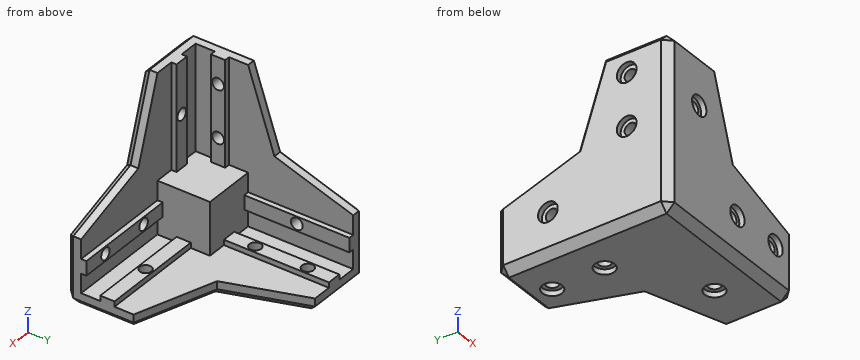
```python
from build123d import *

# Parameters (mm, degrees)
F1_DEPTH  = 6
F3_DEPTH  = 20
F5_DEPTH  = 40
F7_DEPTH  = 60
F9_DEPTH  = 2
F11_DEPTH = 2
F13_DEPTH = 2
F14_R     = 2.25
F15_DEPTH = 8
F16_R     = 2.25
F17_DEPTH = 8
F18_R     = 2.25
F19_DEPTH = 8
F20_R     = 3.75
F21_DEPTH = 2
F22_R     = 3.75
F23_DEPTH = 2
F24_R     = 3.75
F25_DEPTH = 2
F26_W     = 20
F26_H     = 20
F27_DEPTH = 20
F29_DEPTH = 6
F31_DEPTH = 6
F33_DEPTH = 6
F34_SIZE  = 3


with BuildPart() as f1:
    # F0 (on Top) → F1 (new body)
    with BuildSketch(Plane.XY):
        Polygon((0, 66), (0, 0), (66, 0), (66, 26), (26, 26), (26, 66), align=None)
    extrude(amount=F1_DEPTH)

    # F2 (on face) → F3 (join)
    with BuildSketch(Plane.XY.offset(6)):
        Polygon((6, 66), (0, 66), (0, 0), (66, 0), (66, 6), (6, 6), align=None)
    extrude(amount=F3_DEPTH)

    # F4 (on face) → F5 (join)
    with BuildSketch(Plane.XY.offset(26)):
        Polygon((6, 6), (6, 26), (0, 26), (0, 0), (26, 0), (26, 6), align=None)
    extrude(amount=F5_DEPTH)

    # F6 (on face) → F7 (join)
    with BuildSketch(Plane.XY.offset(6)):
        Polygon((13.29, 6), (16, 6), (18.71, 6), (18.71, 8), (13.29, 8), align=None)
        Polygon((6, 18.71), (6, 16), (6, 13.29), (8, 13.29), (8, 18.71), align=None)
    extrude(amount=F7_DEPTH)

    # F8 (on face) → F9 (join)
    with BuildSketch(Plane.XY.offset(6)):
        Polygon((66, 13.29), (66, 16), (66, 18.71), (26, 18.71), (26, 13.29), align=None)
        Polygon((18.71, 66), (16, 66), (13.29, 66), (13.29, 26), (18.71, 26), align=None)
    extrude(amount=F9_DEPTH)

    # F10 (on face) → F11 (join)
    with BuildSketch(Plane(origin=(0, 6, 0), x_dir=(-1, 0, 0), z_dir=(0, 1, 0))):
        Polygon((-66, 18.71), (-66, 16), (-66, 13.29), (-26, 13.29), (-26, 16), (-26, 18.71), align=None)
    extrude(amount=F11_DEPTH)

    # F12 (on face) → F13 (join)
    with BuildSketch(Plane.YZ.offset(6)):
        Polygon((66, 13.29), (66, 16), (66, 18.71), (26, 18.71), (26, 13.29), align=None)
    extrude(amount=F13_DEPTH)

    # F14 (on face) → F15 (cut, through all)
    with BuildSketch(Plane.XZ):
        with Locations((56, 16)):
            Circle(F14_R)
        with Locations((16, 46)):
            Circle(F14_R)
        with Locations((36, 16)):
            Circle(F14_R)
    extrude(amount=-F15_DEPTH, mode=Mode.SUBTRACT)

    # F16 (on face) → F17 (cut, through all)
    with BuildSketch(Plane(origin=(0, 0, 0), x_dir=(0, -1, 0), z_dir=(-1, 0, 0))):
        with Locations((-16, 56)):
            Circle(F16_R)
        with Locations((-46, 16)):
            Circle(F16_R)
        with Locations((-16, 36)):
            Circle(F16_R)
    extrude(amount=-F17_DEPTH, mode=Mode.SUBTRACT)

    # F18 (on face) → F19 (cut, through all)
    with BuildSketch(Plane(origin=(0, 0, 0), x_dir=(1, 0, 0), z_dir=(0, 0, -1))):
        with Locations((46, -16)):
            Circle(F18_R)
        with Locations((16, -56)):
            Circle(F18_R)
        with Locations((16, -36)):
            Circle(F18_R)
    extrude(amount=-F19_DEPTH, mode=Mode.SUBTRACT)

    # F20 (on face) → F21 (cut)
    with BuildSketch(Plane.XZ):
        with Locations((16, 46)):
            Circle(F20_R)
        with Locations((36, 16)):
            Circle(F20_R)
        with Locations((56, 16)):
            Circle(F20_R)
    extrude(amount=-F21_DEPTH, mode=Mode.SUBTRACT)

    # F22 (on face) → F23 (cut)
    with BuildSketch(Plane(origin=(0, 0, 0), x_dir=(0, -1, 0), z_dir=(-1, 0, 0))):
        with Locations((-16, 56)):
            Circle(F22_R)
        with Locations((-46, 16)):
            Circle(F22_R)
        with Locations((-16, 36)):
            Circle(F22_R)
    extrude(amount=-F23_DEPTH, mode=Mode.SUBTRACT)

    # F24 (on face) → F25 (cut)
    with BuildSketch(Plane(origin=(0, 0, 0), x_dir=(1, 0, 0), z_dir=(0, 0, -1))):
        with Locations((16, -56)):
            Circle(F24_R)
        with Locations((46, -16)):
            Circle(F24_R)
        with Locations((16, -36)):
            Circle(F24_R)
    extrude(amount=-F25_DEPTH, mode=Mode.SUBTRACT)

    # F26 (on face) → F27 (join)
    with BuildSketch(Plane.XY.offset(6)):
        with Locations((16, 16)):
            Rectangle(F26_W, F26_H)
    extrude(amount=F27_DEPTH)

    # F28 (on face) → F29 (join)
    with BuildSketch(Plane.XZ):
        Polygon((36, 36), (26, 66), (26, 26), (66, 26), align=None)
    extrude(amount=-F29_DEPTH)

    # F30 (on face) → F31 (join)
    with BuildSketch(Plane(origin=(0, 0, 0), x_dir=(0, -1, 0), z_dir=(-1, 0, 0))):
        Polygon((-26, 26), (-26, 66), (-36, 36), (-66, 26), align=None)
    extrude(amount=-F31_DEPTH)

    # F32 (on face) → F33 (join)
    with BuildSketch(Plane(origin=(0, 0, 0), x_dir=(1, 0, 0), z_dir=(0, 0, -1))):
        Polygon((36, -36), (66, -26), (26, -26), (26, -66), align=None)
    extrude(amount=-F33_DEPTH)

    # F34
    f34_edges = [f1.edges().sort_by_distance(p)[0] for p in [
        (33, 0, 0),
        (66, 13, 0),
        (51, 31, 0),
        (31, 51, 0),
        (13, 66, 0),
        (0, 33, 0),
        (0, 66, 13),
        (0, 51, 31),
        (0, 31, 51),
        (0, 13, 66),
        (0, 0, 33),
        (66, 0, 13),
        (51, 0, 31),
        (31, 0, 51),
        (13, 0, 66),
    ]]
    chamfer(f34_edges, length=F34_SIZE)


solid = f1.part
```
Verification items for the finished model (mm, model axes). Round coordinates to 2 decimals unless told otherwise and drop trailing zeros. Write each loop counter-clockwise with the first axis right and the second up, starting at its lowest first coordinate (ties: lowest second). Pieces come first, ordered by that corner, then holes. Notation, with made-up numbers: (54.5, 84.25) - (61.5, 84.25) arc R16 cw to (61.5, 104.25) - close; hole circle Ø9 at (82, 20.5). An arc over 180 degrees is marked (long way). Answer as a JSON object with one key per item and string values. Group by question number.
Q1. Section check A-A, the plane x = 46. Enter the section's corners in (y, z), plus the area to 3 significant figures.
Q2. Thickness scan on line 1 (Y direction, x = 55.5, z = 7); line 2 (Z direction, x = 1.2, y = 16); line 3 (Z direction, x = 37.5, y = 6.5). Record the ranges inside material, lowest first.
Q3. Go/stop test with flat-tipped pins: pin 1 Ø7 at (x, z) = (36, 16) entering from -Y; pin 2 Ø6 at (x, y) = (48, 8) entering from +Z; pin 3 Ø6 at (x, z) = (17, 49.5) entering from +Y. Record where each tip stops, or that it passes through.
Q4. Section check C-C, the plane z = 5. Enter the section's corners in (x, y), plus the area to 3 significant figures.
Q5. Section check D-D, the plane x = 16. Give the number of separate pieces and of enclosed holes in the cut face, plus the area to 3 significant figures.
Found:
{
 "1": {"outline": "(0, 3) - (3, 0) - (12.25, 0) - (12.25, 2) - (13.75, 2) - (13.75, 8) - (13.29, 8) - (13.29, 6) - (6, 6) - (6, 13.29) - (8, 13.29) - (8, 18.71) - (6, 18.71) - (6, 32.67) - (3, 32.67) - (0, 29.5) - close; (18.25, 2) - (19.75, 2) - (19.75, 0) - (29.5, 0) - (32.67, 3) - (32.67, 6) - (18.71, 6) - (18.71, 8) - (18.25, 8) - close", "area": "322 mm^2"},
 "2": {"line 1": "y = 0 to 6, 13.29 to 18.71", "line 2": "z = 1.8 to 32.25, 39.75 to 52.25, 59.75 to 64.2", "line 3": "z = 0 to 6, 13.29 to 14.32, 17.68 to 18.71"},
 "3": {"pin 1": "stops at y = 2", "pin 2": "stops at z = 32.75", "pin 3": "stops at y = 8"},
 "4": {"outline": "(0, 3) - (3, 0) - (63, 0) - (66, 3) - (66, 26) - (36, 36) - (26, 66) - (3, 66) - (0, 63) - close; hole circle Ø4.5 at (16, 36); hole circle Ø4.5 at (16, 56); hole circle Ø4.5 at (46, 16)", "area": "3,090 mm^2"},
 "5": {"separate pieces": "4", "enclosed holes": "0", "area": "1,180 mm^2"}
}
